The listing builds one solid part. Answer for the finished solid, in the listing's coordinates (mm). Face numbers are marked on the shaded views. A direction names the side the tool comes from. Give positions to 0.01 mm unless a question says otherwise; leave off trailing zeros. Write each loop counter-clockwise with the first axis right and the second up, starting at its lowest first coordinate (ties: lowest second). Pieces come first, ordered by that corner, then holes. Notation, with made-up numbers: (12, 57) -> (59, 57) arc R9 cw to (59, 65) -> close; hole circle Ø8 at (4.5, 65). An arc over 180 degrees is marked (long way). Put each result on its own line as item: value. Start each with the question number.
1) A cutting plane is placed at D-D (x = -15). Write down the section's boundary in (y, z), then the cut area to 3 significant figures.
2) A cutting plane is placed at B-B (z = 3.5). Give the number of separate pieces and of enclosed holes in the cut face, then the cut area to 3 significant figures.
3) A cutting plane is placed at C-C (y = 1.5). Write down the section's boundary in (x, z).
4) For the marked faces 4, 5 and 6, determine the directions among +Z, -Z, +X, -X, +Y, -Y from which every point of the face is accessible in a straight line to the end or side of a thin tool.
5) Flat-ended cylindrical pins translate along their axes: pin 1 Ø1.5 at (x, z) = (16, 4.5) entering from -Y; pin 2 Ø5 at (x, y) = (14.5, 8.5) entering from +Z; pin 3 Ø1.5 at (x, z) = (5.5, 3.5) entering from +Y. Find the tip coordinate at first contact, or state that the pin passes through.
6) For a pull along Y with two mould halves and no side action, classify the marked faces 1, 2 and 3 as released by +Y, released by -Y, zero draft, split by the parting line, or undercut.
7) A cutting plane is placed at A-A (x = 0). Write down the section's boundary in (y, z).
8) Find the intervals of material crossed by line 1 along Y through (x, z) = (0, 0.5); line 2 along Y through (x, z) = (1.5, 5.75); line 3 along X through (y, z) = (-15.5, 3), in increasing order. Write a range as from..to.
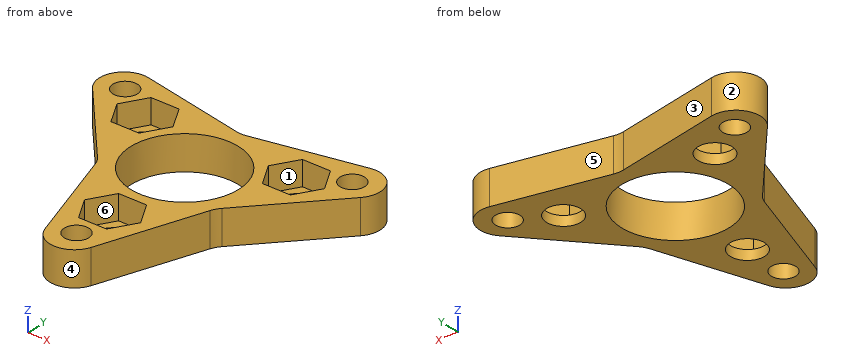
from build123d import *

# Parameters (mm, degrees)
F0_R     = 2.5
F0_R_2   = 11
F1_DEPTH = 7
F0_R_3   = 3.5
F2_DEPTH = 2
F3_R     = 5


# Not quite as in the source:
# - a feature names something its author has since deleted; it is built from what else it names


with BuildPart() as f1:
    # F0 (on Top) → F1 (new body)
    with BuildSketch(Plane.XY):
        Polygon((0, 14), (-37.5, 21.6506350946), (-12.124355653, -7), (0, -43.3012701892), (12.124355653, -7), (37.5, 21.6506350946), align=None)
        with Locations((0, -27)):
            Circle(F0_R, mode=Mode.SUBTRACT)
        Polygon((2.8867513459, -13), (5.7735026919, -18), (2.8867513459, -23), (-2.8867513459, -23), (-5.7735026919, -18), (-2.8867513459, -13), align=None, mode=Mode.SUBTRACT)
        with Locations((-23.3826859022, 13.5)):
            Circle(F0_R, mode=Mode.SUBTRACT)
        Polygon((-12.7017059222, 4), (-18.4752086141, 4), (-21.36195996, 9), (-18.4752086141, 14), (-12.7017059222, 14), (-9.8149545762, 9), align=None, mode=Mode.SUBTRACT)
        Circle(F0_R_2, mode=Mode.SUBTRACT)
        Polygon((21.36195996, 9), (18.4752086141, 4), (12.7017059222, 4), (9.8149545762, 9), (12.7017059222, 14), (18.4752086141, 14), align=None, mode=Mode.SUBTRACT)
        with Locations((23.3826859022, 13.5)):
            Circle(F0_R, mode=Mode.SUBTRACT)
    extrude(amount=F1_DEPTH)

    # F0 (on Top) → F2 (join)
    with BuildSketch(Plane.XY):
        Polygon((-21.36195996, 9), (-18.4752086141, 4), (-12.7017059222, 4), (-9.8149545762, 9), (-12.7017059222, 14), (-18.4752086141, 14), align=None)
        with Locations((-15.5884572681, 9)):
            Circle(F0_R_3, mode=Mode.SUBTRACT)
        Polygon((2.8867513459, -23), (5.7735026919, -18), (2.8867513459, -13), (-2.8867513459, -13), (-5.7735026919, -18), (-2.8867513459, -23), align=None)
        with Locations((0, -18)):
            Circle(F0_R_3, mode=Mode.SUBTRACT)
        Polygon((12.7017059222, 4), (18.4752086141, 4), (21.36195996, 9), (18.4752086141, 14), (12.7017059222, 14), (9.8149545762, 9), align=None)
        with Locations((15.5884572681, 9)):
            Circle(F0_R_3, mode=Mode.SUBTRACT)
    extrude(amount=F2_DEPTH)

    # F3
    f3_edges = [f1.edges().sort_by_distance(p)[0] for p in [
        (37.5, 21.650635, 3.5),
        (-37.5, 21.650635, 3.5),
        (0, -43.30127, 3.5),
        (-12.124356, -7, 3.5),
        (0, 14, 3.5),
        (12.124356, -7, 3.5),
    ]]
    fillet(f3_edges, radius=F3_R)


solid = f1.part
Reply:
1. outline: (-3.75, 0) -> (5.55, 0) -> (5.55, 2) -> (4, 2) -> (4, 7) -> (-3.75, 7) -> close; (12.45, 0) -> (17.06, 0) -> (17.06, 7) -> (14, 7) -> (14, 2) -> (12.45, 2) -> close
1. area: 81.9 mm2
2. separate pieces: 1
2. enclosed holes: 7
2. area: 745 mm2
3. outline: (-19.65, 0) -> (-10.9, 0) -> (-10.9, 7) -> (-19.65, 7) -> close; (10.9, 0) -> (19.65, 0) -> (19.65, 7) -> (10.9, 7) -> close
4. face 4: +Z, -Z, -Y
4. face 5: +Z, -Z, +Y
4. face 6: +Z
5. pin 1: stops at y = -3.47
5. pin 2: stops at z = 2
5. pin 3: stops at y = 15.28
6. face 1: undercut
6. face 2: split by the parting line
6. face 3: released by +Y
7. outline: (-32.52, 0) -> (-29.5, 0) -> (-29.5, 7) -> (-32.52, 7) -> close; (-24.5, 0) -> (-21.5, 0) -> (-21.5, 2) -> (-23, 2) -> (-23, 7) -> (-24.5, 7) -> close; (-14.5, 0) -> (-11, 0) -> (-11, 7) -> (-13, 7) -> (-13, 2) -> (-14.5, 2) -> close; (11, 0) -> (14.1, 0) -> (14.1, 7) -> (11, 7) -> close
8. line 1: y = -32.52..-29.5, -24.5..-21.5, -14.5..-11, 11..14.1
8. line 2: y = -32.29..-29, -25..-23, -13..-10.9, 10.9..14.31
8. line 3: x = -9.29..-4.33, 4.33..9.29
